Here's the drawing with two shaded views (mm, measured from the low corner). I have some questions. A direction names the side the tool comes from. Coordinates: 2 decimals unless noted, no trailing zeros. Loops run counter-clockwise (first coordinate to the right, second up) from the corner with the lowest first, then second, coordinate; pieces in that order, holes last.
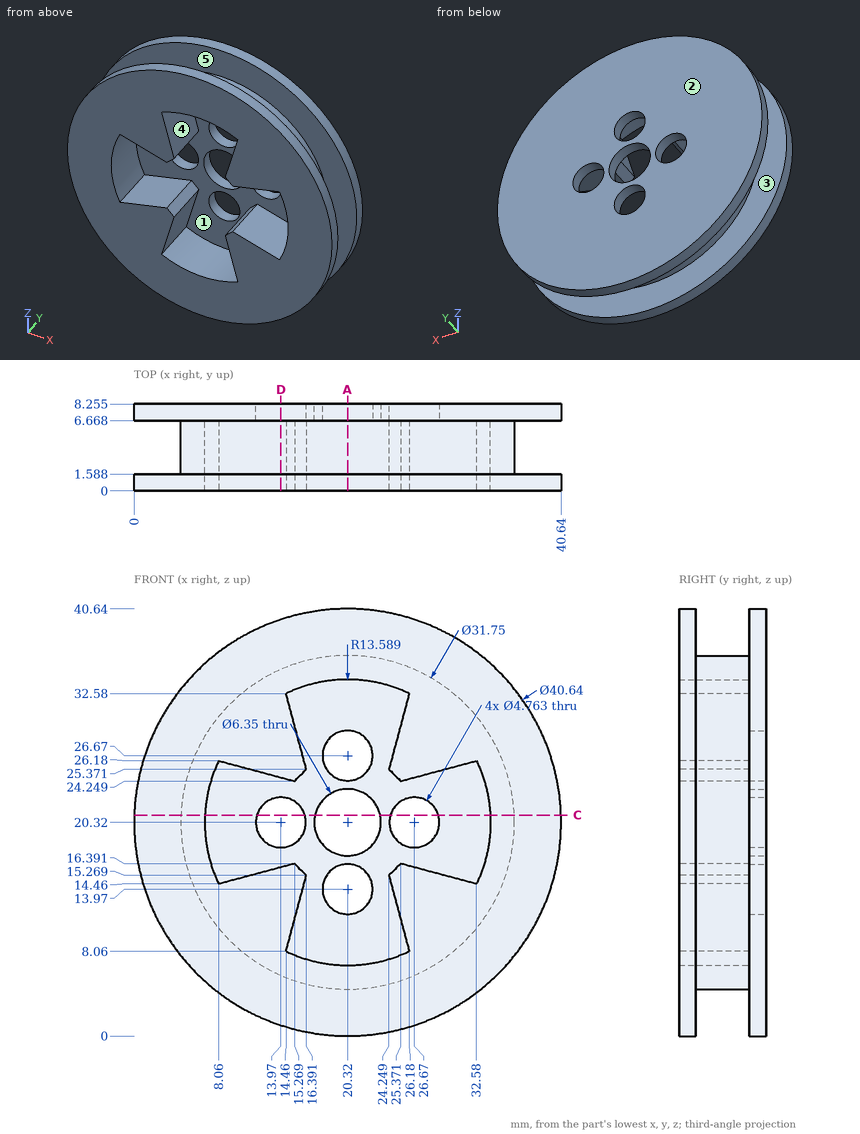
(1) If we mould it in two halves opening along Z, with no side actions, what happens to the marked faces 4 and 5? For each: released by +Z, released by -Z, zero draft, split by the parting line, or undercut.
Check values:
face 4: undercut
face 5: zero draft
(2) I want a section at D-D on x = 13.97. Write out the boundary of the cut face in (y, z) (1 decimal).
Check values:
outline: (0, 1) - (1.6, 1) - (1.6, 5.8) - (6.7, 5.8) - (6.7, 1) - (8.3, 1) - (8.3, 17.9) - (6.7, 17.9) - (6.7, 16) - (0, 16) - close; (0, 24.6) - (6.7, 24.6) - (6.7, 22.7) - (8.3, 22.7) - (8.3, 39.6) - (6.7, 39.6) - (6.7, 34.9) - (1.6, 34.9) - (1.6, 39.6) - (0, 39.6) - close
(3) I want a section at C-C on z = 21. Write out the boundary of the cut face in (x, y) (1 decimal).
Check values:
outline: (0, 0) - (6.7, 0) - (6.7, 6.7) - (11.7, 6.7) - (11.7, 8.3) - (0, 8.3) - (0, 6.7) - (4.5, 6.7) - (4.5, 1.6) - (0, 1.6) - close; (16.3, 6.7) - (17.2, 6.7) - (17.2, 8.3) - (16.3, 8.3) - close; (23.4, 6.7) - (24.4, 6.7) - (24.4, 8.3) - (23.4, 8.3) - close; (29, 6.7) - (33.9, 6.7) - (33.9, 0) - (40.6, 0) - (40.6, 1.6) - (36.2, 1.6) - (36.2, 6.7) - (40.6, 6.7) - (40.6, 8.3) - (29, 8.3) - close
(4) I'm going to push flat-ended pins straight in: pin 1 (6 mm diameter, centred on x = 26.67, z = 20.32, fed in from -Y); pin 2 (1 mm diameter, centred on x = 19.5, y = 1.5, fed in from -Z); pin 3 (4 mm diameter, centred on x = 19, y = 1.5, fed in from +Z); pin 4 (3 mm diameter, centred on x = 20.32, z = 13.97, fed in from -Y). Where does each tip first touch, or does it pass through?
Check values:
pin 1: stops at y = 6.67
pin 2: stops at z = 0
pin 3: stops at z = 40.64
pin 4: passes through
(5) If I drill on probe 1 along Z at (x, y) = (20.32, 7.35) (1 decimal); probe 2 along Y at (x, z) = (2, 18) (1 decimal); probe 3 along Y at (x, z) = (17, 32) (1 decimal), over which ranges is the centre line in solid material (lowest first)?
Check values:
probe 1: z = 0 to 11.6, 16.4 to 17.1, 23.5 to 24.3, 29.1 to 40.6
probe 2: y = 0 to 1.6, 6.7 to 8.3
probe 3: y = 6.7 to 8.3
(6) I want a section at A-A on x = 20.32. Write out the boundary of the cut face in (y, z) (1 decimal).
Check values:
outline: (0, 0) - (1.6, 0) - (1.6, 4.4) - (6.7, 4.4) - (6.7, 0) - (8.3, 0) - (8.3, 11.6) - (6.7, 11.6) - (6.7, 6.7) - (0, 6.7) - close; (0, 33.9) - (6.7, 33.9) - (6.7, 29.1) - (8.3, 29.1) - (8.3, 40.6) - (6.7, 40.6) - (6.7, 36.2) - (1.6, 36.2) - (1.6, 40.6) - (0, 40.6) - close; (6.7, 16.4) - (8.3, 16.4) - (8.3, 17.1) - (6.7, 17.1) - close; (6.7, 23.5) - (8.3, 23.5) - (8.3, 24.3) - (6.7, 24.3) - close
(7) Which directions (+Z, -Z, +X, -X, +Y, -Y) give clear straight access to the entire face, cutting with the end or side of a thin tool? Please do the marked faces 1, 2 and 3.
Check values:
face 1: -Y
face 2: +Z, -Z, +X, -X, +Y
face 3: none
